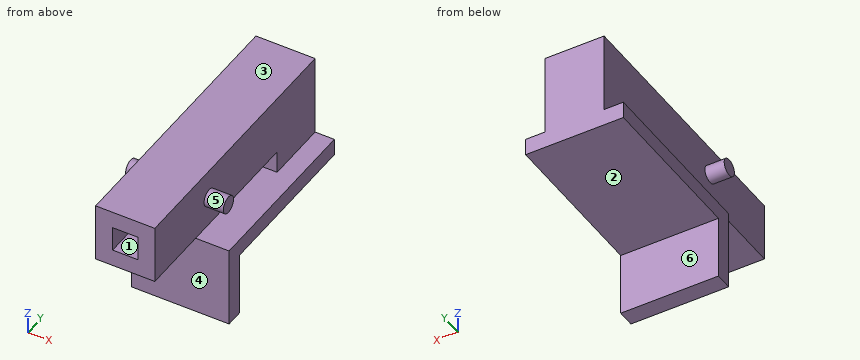
from build123d import *

# Parameters (mm, degrees)
SKETCH1_W           = 10.442861366
SKETCH1_H           = 47.180745659
BOSS_EXTRUDE1_DEPTH = 10.4
SKETCH2_W           = 4.442861366
SKETCH2_H           = 4.4
CUT_EXTRUDE1_DEPTH  = 25
WRAP1_START         = 6.090842934
WRAP1_OUTLINE_R     = 1.5
WRAP1_DEPTH         = 3.4
WRAP2_START         = -7.752018432
WRAP2_OUTLINE_R     = 1.5
WRAP2_DEPTH         = 3.4
SKETCH9_W           = 14.4
SKETCH9_H           = 11.180745659
BOSS_EXTRUDE2_DEPTH = 10.442861366
SKETCH10_W          = 17.242861366
SKETCH10_H          = 28
BOSS_EXTRUDE3_DEPTH = 3
SKETCH11_W          = 17.242861366
SKETCH11_H          = 14.30503792
BOSS_EXTRUDE4_DEPTH = 3


# Read off the part's stored shape, not the designer's step: Wrap1, Wrap2
with BuildPart() as part:
    # Sketch1 → Boss-Extrude1 (new body)
    with BuildSketch(Plane.XY):
        with Locations((0.869412251, 15.507053004)):
            Rectangle(SKETCH1_W, SKETCH1_H)
    extrude(amount=-BOSS_EXTRUDE1_DEPTH)

    # Sketch2 → Cut-Extrude1 (cut)
    with BuildSketch(Plane(origin=(0, -8.083319826, 0), x_dir=(-1, 0, 0), z_dir=(0, -1, 0))):
        with Locations((-0.869412251, 5.2)):
            Rectangle(SKETCH2_W, SKETCH2_H)
    extrude(amount=-CUT_EXTRUDE1_DEPTH, mode=Mode.SUBTRACT)

    # Wrap1 outline → Wrap1 (add)
    with BuildSketch(Plane(origin=(0, 0, 0), x_dir=(0, 0, -1), z_dir=(1, 0, 0)).offset(WRAP1_START)):
        with Locations((5.2, 7.916680174)):
            Circle(WRAP1_OUTLINE_R)
    extrude(amount=WRAP1_DEPTH)

    # Wrap2 outline → Wrap2 (add)
    with BuildSketch(Plane(origin=(0, 0, 0), x_dir=(0, 0, -1), z_dir=(1, 0, 0)).offset(WRAP2_START)):
        with Locations((5.2, 7.916680174)):
            Circle(WRAP2_OUTLINE_R)
    extrude(amount=WRAP2_DEPTH)

    # Sketch9 → Boss-Extrude2 (add)
    with BuildSketch(Plane(origin=(6.090842934, 0, 0), x_dir=(0, 0, -1), z_dir=(1, 0, 0))):
        with Locations((7.2, 33.507053004)):
            Rectangle(SKETCH9_W, SKETCH9_H)
    extrude(amount=-BOSS_EXTRUDE2_DEPTH)

    # Sketch10 → Boss-Extrude3 (add)
    with BuildSketch(Plane(origin=(0, 0, -14.4), x_dir=(-1, 0, 0), z_dir=(0, 0, -1))):
        with Locations((-0.869412251, 25.097425833)):
            Rectangle(SKETCH10_W, SKETCH10_H)
    extrude(amount=BOSS_EXTRUDE3_DEPTH)

    # Sketch11 → Boss-Extrude4 (add)
    with BuildSketch(Plane(origin=(0, 11.097425833, 0), x_dir=(-1, 0, 0), z_dir=(0, -1, 0))):
        with Locations((-0.869412251, 21.55251896)):
            Rectangle(SKETCH11_W, SKETCH11_H)
    extrude(amount=BOSS_EXTRUDE4_DEPTH)


solid = part.part
Could you check a few things on this model? Use its own coordinates, in mm. Face numbers are marked on the shaded views. A direction names the side the tool comes from. Give positions to 0.01 mm unless a question says otherwise; leave off trailing zeros. Loops run counter-clockwise (first coordinate to the right, second up) from the corner with the lowest first, then second, coordinate; pieces in that order, holes last. Notation, with made-up numbers: (7.25, 33.25) -> (23.25, 33.25) arc R33 cw to (23.25, 63.25) -> close; hole circle Ø11 at (85, 66.5). An arc over 180 degrees is marked (long way). Return JSON: item names as keys, results as strings.
Item 1: If we section it at B-B on z = -5.2: List the corners of the cut face in (x, y) for me, plus the area to 3 significant figures.
Geometry results:
{"outline": "(-7.75, 6.42) -> (-4.35, 6.42) -> (-4.35, -8.08) -> (-1.35, -8.08) -> (-1.35, 16.92) -> (3.09, 16.92) -> (3.09, -8.08) -> (6.09, -8.08) -> (6.09, 6.42) -> (9.49, 6.42) -> (9.49, 9.42) -> (6.09, 9.42) -> (6.09, 39.1) -> (-4.35, 39.1) -> (-4.35, 9.42) -> (-7.75, 9.42) -> close", "area": "402 mm²"}
Item 2: If we section it at C-C on x = 0.5: List the corners of the cut face in (y, z) for me, plus the area to 3 significant figures.
Geometry results:
{"outline": "(-8.08, -10.4) -> (27.92, -10.4) -> (27.92, -14.4) -> (8.1, -14.4) -> (8.1, -28.71) -> (11.1, -28.71) -> (11.1, -17.4) -> (39.1, -17.4) -> (39.1, 0) -> (-8.08, 0) -> (-8.08, -3) -> (16.92, -3) -> (16.92, -7.4) -> (-8.08, -7.4) -> close", "area": "552 mm²"}
Item 3: We'd pull the mould along Z, two halves only. Please class the marked faces 1, 2 and 3: +Z half, -Z half, draft (parallel to the pull), parting line (faces both ways), or undercut.
Geometry results:
{"face 1": "undercut", "face 2": "-Z half", "face 3": "+Z half"}
Item 4: Which directions (+Z, -Z, +X, -X, +Y, -Y) give clear straight access to the entire face, cutting with the end or side of a thin tool? Please do the marked faces 4, 5 and 6.
Geometry results:
{"face 4": "-Z, +X, -X, -Y", "face 5": "+X", "face 6": "-Z, +X, -X, +Y"}
Item 5: If we section it at D-D on y = 2: List the corners of the cut face in (x, z) for me.
Geometry results:
{"outline": "(-4.35, -10.4) -> (6.09, -10.4) -> (6.09, 0) -> (-4.35, 0) -> close; hole (-1.35, -7.4) -> (3.09, -7.4) -> (3.09, -3) -> (-1.35, -3) -> close"}
Item 6: I need wall thicknesses on L1, parallel to Z at x = 3.5, y = 18.5; L2, parallel to Z at x = 2.5, y = 14; L3, parallel to Z at x = 5.25, y = 37. Which ranges of each line are inside material? Lowest first, please. Write a range as from..to.
Geometry results:
{"L1": "z = -17.4..-14.4, -10.4..0", "L2": "z = -17.4..-14.4, -10.4..-7.4, -3..0", "L3": "z = -17.4..0"}
Item 7: I'm going to push flat-ended pins straight in: pin 1 (4.5 mm diameter, centred on y = 24, z = -6, fed in from +X); pin 2 (16 mm diameter, centred on y = 19.5, z = -4, fed in from -X); pin 3 (2 mm diameter, centred on x = 1.5, y = 2.5, fed in from -Z). Where does each tip first touch, or does it pass through?
Geometry results:
{"pin 1": "stops at x = 6.09", "pin 2": "stops at x = -4.35", "pin 3": "stops at z = -10.4"}
Item 8: If we section it at A-A on y = 21: List the corners of the cut face in (x, z) for me.
Geometry results:
{"outline": "(-7.75, -17.4) -> (9.49, -17.4) -> (9.49, -14.4) -> (-7.75, -14.4) -> close; (-4.35, -10.4) -> (6.09, -10.4) -> (6.09, 0) -> (-4.35, 0) -> close"}
